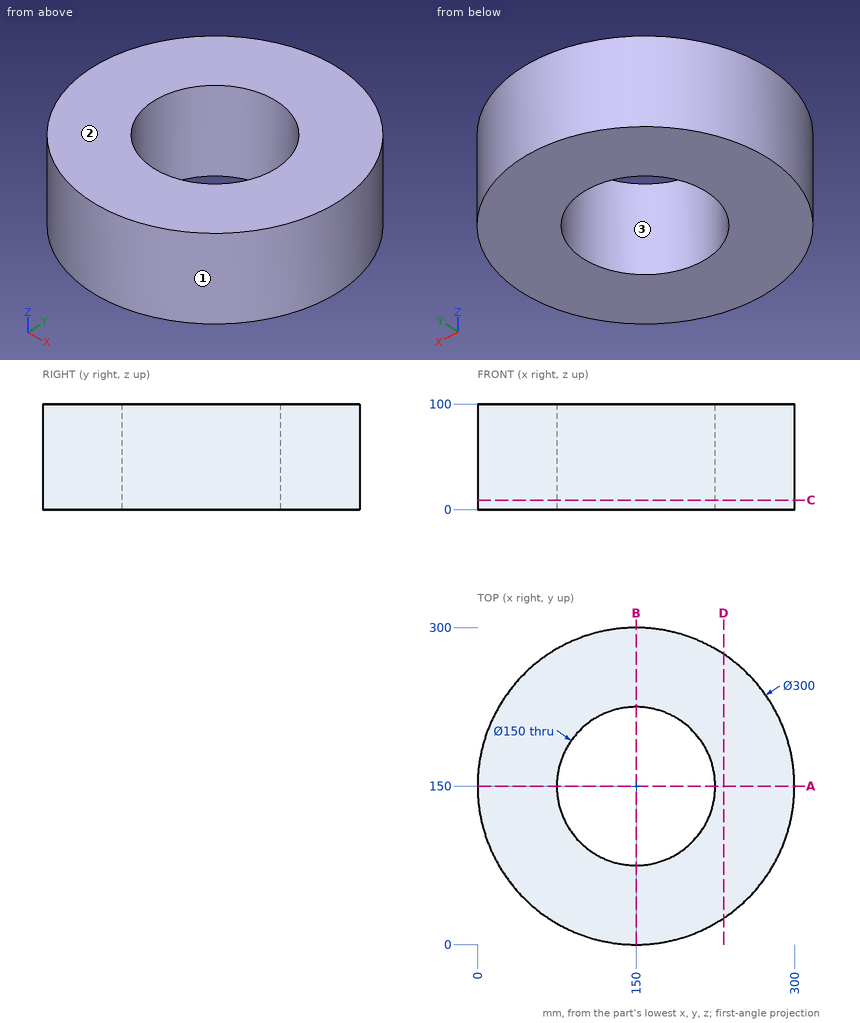
Job drawing, mm, ordinate dimensions from the low corner. One solid piece. Round coordinates to 2 decimals unless told otherwise and drop trailing zeros. Write each loop counter-clockwise with the first axis right and the second up, starting at its lowest first coordinate (ties: lowest second). Pieces come first, ordered by that corner, then holes. Notation, with made-up numbers: M 22.25,-29 L 52.25,-29 A16 ccw 52.25,-23 Z; hole C -24.75,-22.75 d5. An arc over 180 degrees is marked long. Return JSON: item names as keys, results as strings. Group by question number.
(1) Saw through at A-A on y = 150. Write the cut outline in (x, z), then the cut area to 3 significant figures.
(2) Pin check, flat tips, straight feed: pin 1 Ø4 at (y, z) = (187.5, 81.5) entering from +X; pin 2 Ø5 at (x, z) = (66, 82.5) entering from +Y; pin 3 Ø5 at (y, z) = (208, 37) entering from -X. Stop position of each tip, or through.
(3) Drill centre lines: probe 1 along X at (y, z) = (147.5, 85); probe 2 along Y at (x, z) = (150, 71); probe 3 along X at (y, z) = (204, 13.5). Where is each one in solid material? Low to high.
(4) Saw through at C-C on z = 9. Write the cut outline in (x, y).
(5) Saw through at D-D on x = 233. Write the cut outline in (y, z), then the cut area to 3 significant figures.
(6) Two-plate mould, pull along Y, no slides. Class the marked faces 1, 2 and 3: +Y half, -Y half, draft (parallel to the pull), parting line (faces both ways), or undercut.
Returned:
{
 "1": {"outline": "M 0,0 L 75,0 L 75,100 L 0,100 Z; M 225,0 L 300,0 L 300,100 L 225,100 Z", "area": "15,000 mm²"},
 "2": {"pin 1": "x = 295.74", "pin 2": "y = 275.93", "pin 3": "x = 10.65"},
 "3": {"probe 1": "0.02 to 75.04, 224.96 to 299.98", "probe 2": "0 to 75, 225 to 300", "probe 3": "10.06 to 97.95, 202.05 to 289.94"},
 "4": {"outline": "C 150,150 d300; hole C 150,150 d150"},
 "5": {"outline": "M 25.06,0 L 274.94,0 L 274.94,100 L 25.06,100 Z", "area": "25,000 mm²"},
 "6": {"face 1": "parting line", "face 2": "draft", "face 3": "undercut"}
}
